Input: part model. Units: mm. Frame: model coordinates. A direction names the side the tool comes from. Round coordinates to 2 decimals unless told otherwise and drop trailing zeros. Loops run counter-clockwise (first coordinate to the right, second up) from the corner with the lowest first, then second, coordinate; pieces in that order, holes last. Notation, with made-up numbers: (24, 12.5) - (53, 12.5) arc R15 ccw to (53, 19.5) - close; hole circle Ø7 at (18, 39.25). An arc over 180 degrees is marked (long way). One line per question, with ' | ' between items. Start each with the question number.
Item 1: Set-up query: faces 1 (the face through (-6.1, 1.85, 0.5)), 2 (the face through (-5, 0, 0)), 3 (the face through (-6.2, -1.85, 0.5)), 4 (the face through (-9.5, 0, 0.5)), 5 (the face through (-1, 0, 1)). Return all of +Z, -Z, +X, -X, +Y, -Y with unobstructed straight access to the full face (end or side cutting, diameter ignored); none if empty.
Item 2: Section C-C, the plane x = -2.25. Return loops of the section in (y, z), plus the area to 3 significant figures.
Item 3: Draft query along X for faces 6 (the face through (2.67, 0.84, 1.58)), 7 (the face through (-12, 0, 0.5)), 8 (the face through (-0.75, 0.03, 0.49)). Return one class per face: pulls with the +X half, pulls with the -X half, needs draft (parallel to the pull), parting line crosses it, or undercut.
Item 4: First-contact query: pin 1 (1 mm diameter, centred on x = 0, y = 0.5, fed in from -Z); pin 2 (1.1 mm diameter, centred on x = -7, y = -0.5, fed in from +Z); pin 3 (0.8 mm diameter, centred on x = -4.5, z = 0.5, fed in from +Y). Flat tips, straight axial feed; report the tip coordinate or a pass-through.
Item 5: Material intervals for line 1 along Y through (x, z) = (0, 0.65); line 2 along Y through (x, z) = (-10, 0.7); line 3 along X through (y, z) = (-2.25, 0.55), sorted ascending.
Item 6: Section D-D, the plane x = -8. Return loops of the section in (y, z).
Item 7: Section A-A, the plane x = -10. Return loops of the section in (y, z), plus the area to 3 significant figures.
```python
from build123d import *

# Parameters (mm, degrees)
SKETCH1_R           = 2.8
BOSS_EXTRUDE1_DEPTH = 3.2
CUT_EXTRUDE1_DEPTH  = 2.2
SKETCH3_R           = 0.75
CUT_EXTRUDE2_DEPTH  = 1
BOSS_EXTRUDE2_DEPTH = 1
CUT_EXTRUDE3_REACH  = 5.2
SKETCH5_R           = 0.5


with BuildPart() as part:
    # Sketch1 → Boss-Extrude1 (new body)
    with BuildSketch(Plane.XY):
        Circle(SKETCH1_R)
    extrude(amount=BOSS_EXTRUDE1_DEPTH)

    # Sketch2 → Cut-Extrude1 (cut)
    with BuildSketch(Plane.XY.offset(3.2)):
        Polygon((0.014651949, 1.985348051), (-0.313876209, 1.636970634), (-0.750714916, 1.833107116), (-0.920917091, 1.385526068), (-1.399561614, 1.399561614), (-1.385526068, 0.920917091), (-1.833107116, 0.750714916), (-1.636970634, 0.313876209), (-1.985348051, -0.014651949), (-1.636970634, -0.343180107), (-1.833107116, -0.780018813), (-1.385526068, -0.950220989), (-1.399561614, -1.428865511), (-0.920917091, -1.414829965), (-0.750714916, -1.862411014), (-0.313876209, -1.666274532), (0.014651949, -2.014651949), (0.343180107, -1.666274532), (0.780018813, -1.862411014), (0.950220989, -1.414829965), (1.428865511, -1.428865511), (1.414829965, -0.950220989), (1.862411014, -0.780018813), (1.666274532, -0.343180107), (2.014651949, -0.014651949), (1.666274532, 0.313876209), (1.862411014, 0.750714916), (1.414829965, 0.920917091), (1.428865511, 1.399561614), (0.950220989, 1.385526068), (0.780018813, 1.833107116), (0.343180107, 1.636970634), align=None)
    extrude(amount=-CUT_EXTRUDE1_DEPTH, mode=Mode.SUBTRACT)

    # Sketch3 → Cut-Extrude2 (cut)
    with BuildSketch(Plane.XY):
        Circle(SKETCH3_R)
    extrude(amount=CUT_EXTRUDE2_DEPTH, mode=Mode.SUBTRACT)

    # Sketch4 → Boss-Extrude2 (add)
    with BuildSketch(Plane.XY):
        with BuildLine():
            Line((-0.75, -1.85), (-0.75, 1.85))
            Line((-0.75, 1.85), (-10.15, 1.85))
            ThreePointArc((-10.15, 1.85), (-12, 0), (-10.15, -1.85))
            Line((-10.15, -1.85), (-0.75, -1.85))
        make_face()
    extrude(amount=BOSS_EXTRUDE2_DEPTH)

    # Sketch5 → Cut-Extrude3 (cut, up to next)
    with BuildSketch(Plane(origin=(0, 0, 0), x_dir=(-1, 0, 0), z_dir=(0, 0, -1)), mode=Mode.PRIVATE) as cut_extrude3_sk1:
        with Locations((10, 0)):
            Circle(SKETCH5_R)
    cut_extrude3_tool1 = extrude(cut_extrude3_sk1.sketch, amount=-CUT_EXTRUDE3_REACH, mode=Mode.PRIVATE) & part.part
    add(cut_extrude3_tool1.solids().sort_by_distance((-10, 0, 0))[0], mode=Mode.SUBTRACT)


solid = part.part
```
Return value:
1) face 1: +Z, -Z, -X, +Y | face 2: -Z, +X, -X, +Y, -Y | face 3: +Z, -Z, -X, -Y | face 4: +Z, -Z | face 5: +Z
2) outline: (-1.85, 0) - (1.85, 0) - (1.85, 1) - (1.67, 1) - (1.67, 3.2) - (-1.67, 3.2) - (-1.67, 1) - (-1.85, 1) - close | area: 11.0 mm2
3) face 6: parting line crosses it | face 7: pulls with the -X half | face 8: undercut
4) pin 1: z = 0 | pin 2: z = 1 | pin 3: y = 1.85
5) line 1: -2.8 to -0.75, 0.75 to 2.8 | line 2: -1.85 to -0.5, 0.5 to 1.85 | line 3: -1.67 to 1.67
6) outline: (-1.85, 0) - (1.85, 0) - (1.85, 1) - (-1.85, 1) - close
7) outline: (-1.85, 0) - (-0.5, 0) - (-0.5, 1) - (-1.85, 1) - close; (0.5, 0) - (1.85, 0) - (1.85, 1) - (0.5, 1) - close | area: 2.70 mm2
